The listing builds one solid part. Answer for the finished solid, in the listing's coordinates (mm). A direction names the side the tool comes from. Give positions to 0.01 mm unless a question says otherwise; leave off trailing zeros. Loops run counter-clockwise (first coordinate to the right, second up) from the corner with the lowest first, then second, coordinate; pieces in that order, holes last. Notation, with made-up numbers: M 81.5,11.5 L 136.5,11.5 A24 cw 136.5,47.5 Z; hole C -16,35.5 d8. An arc over 180 degrees is marked long. Return JSON: item names as keys, results as strings.
from build123d import *

# Parameters (mm, degrees)
F0_R     = 11
F1_DEPTH = 7
F2_R     = 2.5
F4_DEPTH = 25
F5_SIZE  = 0.3


with BuildPart() as f1:
    # F0 (on Top) → F1 (new body)
    with BuildSketch(Plane.XY):
        with BuildLine():
            Line((21.230369, -0.772078), (9.946545, 18.772078))
            ThreePointArc((9.946545, 18.772078), (0, 45), (-9.946545, 18.772078))
            Line((-9.946545, 18.772078), (-21.230369, -0.772078))
            ThreePointArc((-21.230369, -0.772078), (-38.971143, -22.5), (-11.283824, -18))
            Line((-11.283824, -18), (11.283824, -18))
            ThreePointArc((11.283824, -18), (38.971143, -22.5), (21.230369, -0.772078))
        make_face()
        with Locations((-25.980762, -15)):
            Circle(F0_R, mode=Mode.SUBTRACT)
        with Locations((25.980762, -15)):
            Circle(F0_R, mode=Mode.SUBTRACT)
        Circle(F0_R, mode=Mode.SUBTRACT)
        with Locations((0, 30)):
            Circle(F0_R, mode=Mode.SUBTRACT)
    extrude(amount=F1_DEPTH)

    # F2
    f2_edges = [f1.edges().sort_by_distance(p)[0] for p in [
        (11.283824, -18, 3.5),
        (-11.283824, -18, 3.5),
        (-21.230369, -0.772078, 3.5),
        (9.946545, 18.772078, 3.5),
        (21.230369, -0.772078, 3.5),
        (-9.946545, 18.772078, 3.5),
    ]]
    fillet(f2_edges, radius=F2_R)

    # F3 (on face) → F4 (cut)
    with BuildSketch(Plane(origin=(0, 0, 0), x_dir=(1, 0, 0), z_dir=(0, 0, -1))):
        with BuildLine():
            ThreePointArc((7.5, -15), (6.84099, -13.40901), (5.25, -12.75))
            Line((5.25, -12.75), (-5.25, -12.75))
            ThreePointArc((-5.25, -12.75), (-6.84099, -13.40901), (-7.5, -15))
            ThreePointArc((-7.5, -15), (-6.84099, -16.59099), (-5.25, -17.25))
            Line((-5.25, -17.25), (5.25, -17.25))
            ThreePointArc((5.25, -17.25), (6.84099, -16.59099), (7.5, -15))
        make_face()
        with BuildLine():
            ThreePointArc((13.666824, 1.828367), (15.033038, 0.780034), (16.740381, 1.004809))
            ThreePointArc((16.740381, 1.004809), (17.788714, 2.371024), (17.563938, 4.078367))
            Line((17.563938, 4.078367), (12.313938, 13.171633))
            ThreePointArc((12.313938, 13.171633), (10.947724, 14.219966), (9.240381, 13.995191))
            ThreePointArc((9.240381, 13.995191), (8.192048, 12.628976), (8.416824, 10.921633))
            Line((8.416824, 10.921633), (13.666824, 1.828367))
        make_face()
        with BuildLine():
            ThreePointArc((-8.416824, 10.921633), (-8.192048, 12.628976), (-9.240381, 13.995191))
            ThreePointArc((-9.240381, 13.995191), (-10.947724, 14.219966), (-12.313938, 13.171633))
            Line((-12.313938, 13.171633), (-17.563938, 4.078367))
            ThreePointArc((-17.563938, 4.078367), (-17.788714, 2.371024), (-16.740381, 1.004809))
            ThreePointArc((-16.740381, 1.004809), (-15.033038, 0.780034), (-13.666824, 1.828367))
            Line((-13.666824, 1.828367), (-8.416824, 10.921633))
        make_face()
    extrude(amount=-F4_DEPTH, mode=Mode.SUBTRACT)

    # F5
    f5_edges = [f1.edges().sort_by_distance(p)[0] for p in [
        (15.588457, 9, 0),
        (21.414108, -0.143541, 0),
        (10.582744, 18.616932, 0),
        (38.971143, -22.5, 0),
        (0, 45, 0),
        (10.831364, -18.473391, 0),
        (-10.582744, 18.616932, 0),
        (0, -18, 0),
        (-15.588457, 9, 0),
        (-10.831364, -18.473391, 0),
        (-21.414108, -0.143541, 0),
        (-38.971143, -22.5, 0),
        (-36.980762, -15, 0),
        (-9.240381, -13.995191, 0),
        (-11.041824, -6.375, 0),
        (-16.740381, -1.004809, 0),
        (-14.938938, -8.625, 0),
        (14.980762, -15, 0),
        (9.240381, -13.995191, 0),
        (14.938938, -8.625, 0),
        (16.740381, -1.004809, 0),
        (11.041824, -6.375, 0),
        (-11, 0, 0),
        (7.5, 15, 0),
        (0, 17.25, 0),
        (-7.5, 15, 0),
        (0, 12.75, 0),
        (-11, 30, 0),
        (15.588457, 9, 7),
        (21.414108, -0.143541, 7),
        (10.582744, 18.616932, 7),
        (38.971143, -22.5, 7),
        (0, 45, 7),
        (10.831364, -18.473391, 7),
        (-10.582744, 18.616932, 7),
        (0, -18, 7),
        (-15.588457, 9, 7),
        (-10.831364, -18.473391, 7),
        (-21.414108, -0.143541, 7),
        (-38.971143, -22.5, 7),
        (-36.980762, -15, 7),
        (-11.041824, -6.375, 7),
        (-16.740381, -1.004809, 7),
        (-14.938938, -8.625, 7),
        (-9.240381, -13.995191, 7),
        (14.980762, -15, 7),
        (11.041824, -6.375, 7),
        (9.240381, -13.995191, 7),
        (14.938938, -8.625, 7),
        (16.740381, -1.004809, 7),
        (-11, 0, 7),
        (0, 17.25, 7),
        (-7.5, 15, 7),
        (0, 12.75, 7),
        (7.5, 15, 7),
        (-11, 30, 7),
    ]]
    chamfer(f5_edges, length=F5_SIZE)


solid = f1.part
(1) A tool of negligible diameter and unlimited length cuts with its end or side. For faces 1 (the flat face through (15.65, 8.89, 3.46)), 2 (the flat face through (15.522, 8.81, 6.852)), 3 (the flat face through (-15.03, -8.763, 0.152)), 4 (the flat face through (-15.39, 9.04, 6.85)), 5 (the flat face through (10.95, -6.237, 6.848)), from which of +Z, -Z, +X, -X, +Y, -Y can it reach the whole face along a straight path? Write none if from no direction.
Values follow:
{"face 1": "+Z, -Z, +X", "face 2": "+Z, +X", "face 3": "-Z", "face 4": "+Z, -X", "face 5": "+Z"}
(2) The part is cut by section B-B (y = 30). Determine the outline of the cut face in (x, z).
Values follow:
{"outline": "M -15,0.3 L -14.7,0 L -11.3,0 L -11,0.3 L -11,6.7 L -11.3,7 L -14.7,7 L -15,6.7 Z; M 11,0.3 L 11.3,0 L 14.7,0 L 15,0.3 L 15,6.7 L 14.7,7 L 11.3,7 L 11,6.7 Z"}
(3) Determine the mould class of faces 6 (the cylindrical face through (-39.206, -22.078, 3.455)), 7 (the cylindrical face through (-21.394, -0.134, 3.545)), 8 (the flat face through (-14.9, -8.69, 3.46)) for opening direction Y: released by +Y, released by -Y, zero draft, split by the parting line, or undercut.
Values follow:
{"face 6": "split by the parting line", "face 7": "released by +Y", "face 8": "undercut"}
(4) Given pin 1 (2 mm diameter, centred on x = 17.5, z = 4.5, fed in from +Y); pin 2 (1 mm diameter, centred on x = -21.5, z = 2, fed in from +Y); pin 3 (1 mm diameter, centred on x = 23.5, z = 5.5, fed in from -Y), each flat-ended and moving along its own axis, determine where each tip first touches the part or whether it passes through.
Values follow:
{"pin 1": "y = 7.42", "pin 2": "y = 0.09", "pin 3": "y = -29.87"}
(5) The part is cut by section A-A (x = 0). Give the number of separate pieces and of enclosed holes in the cut face, and give its area (3 significant figures).
Values follow:
{"separate pieces": "4", "enclosed holes": "0", "area": "101 mm²"}
(6) Straight lines are drawn through the part: line 1 along Y through (x, z) = (-16.5, 3.75); line 2 along Y through (x, z) = (-3.5, 5.5); line 3 along Y through (x, z) = (-21.5, 3). For each, find the intervals that lie inside material, in ascending order.
Values follow:
{"line 1": "-26.62 to -20.58, -9.42 to -5.92, -0.88 to 7.42", "line 2": "-18 to -10.43, 10.43 to 12.75, 17.25 to 19.57, 40.43 to 44.59", "line 3": "-29.32 to -25.05, -4.95 to -0.18"}
